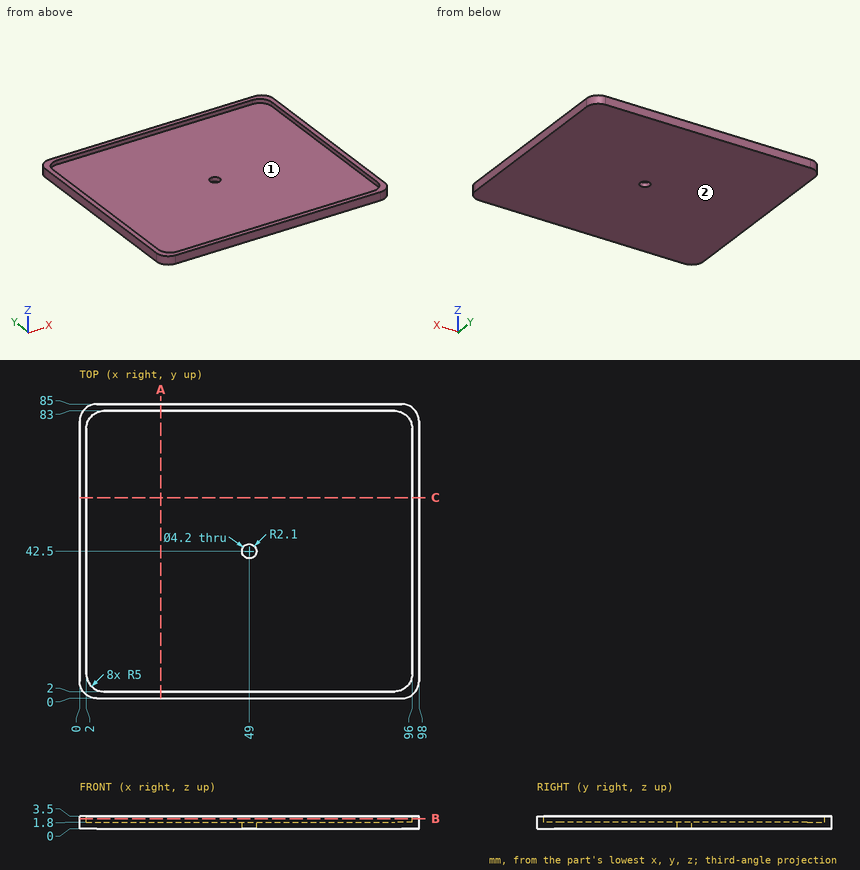
Study the drawing (mm; zero at the part's minimum x, y, z) and answer. Give positions to 0.01 mm unless a question says otherwise; leave off trailing zeros. Order: outer loops, then holes, each group sorted by start corner. A loop starts at its lowest first (then second) coordinate and runs counter-clockwise, first axis right, second up.
1. Each of these flat-tipped pins is pushed along its axis until it touches: P1, Ø1.9, axis at y = 32, z = 2, coming from the -X side; P2, Ø4, axis at x = 34.5, y = 21, coming from the +Z side. Where does it stop, or does it pass through?
Result sheet:
P1: stops at x = 0
P2: stops at z = 1.8
2. Section C-C, the plane y = 58 is taken. Determine the outline of the cut face in (x, z), and give its area (3 significant figures).
Result sheet:
outline: (0, 0) - (98, 0) - (98, 3.5) - (96, 3.5) - (96, 1.8) - (2, 1.8) - (2, 3.5) - (0, 3.5) - close
area: 183 mm2
3. The mould has two halves that part along X. Classify the marked faces 1 and 2: released by +X, released by -X, zero draft, split by the parting line, or undercut.
Result sheet:
face 1: undercut
face 2: zero draft
4. Section A-A, the plane x = 23.5 is taken. Determine the outline of the cut face in (y, z).
Result sheet:
outline: (0, 0) - (85, 0) - (85, 3.5) - (83, 3.5) - (83, 1.8) - (2, 1.8) - (2, 3.5) - (0, 3.5) - close
5. Straight lines are drawn through the part: L1, parallel to X at y = 55.5, z = 3.25; L2, parallel to Y at x = 49, z = 0.5; L3, parallel to X at y = 42.5, z = 0.7. For each, find the intervals that lie inside material, in ascending order.
Result sheet:
L1: x = 0 to 2, 96 to 98
L2: y = 0 to 40.4, 44.6 to 85
L3: x = 0 to 46.9, 51.1 to 98
6. Section B-B, the plane z = 2.85 is taken. Determine the outline of the cut face in (x, y).
Result sheet:
outline: (0, 5) arc R5 ccw to (5, 0) - (93, 0) arc R5 ccw to (98, 5) - (98, 80) arc R5 ccw to (93, 85) - (5, 85) arc R5 ccw to (0, 80) - close; hole (2, 7) arc R5 ccw to (7, 2) - (91, 2) arc R5 ccw to (96, 7) - (96, 78) arc R5 ccw to (91, 83) - (7, 83) arc R5 ccw to (2, 78) - close
